from build123d import *

# Parameters (mm, degrees)
F0_R         = 12.7
F0_R_2       = 6.25
F1_DEPTH     = 4
F3_R         = 12.7
F4_DEPTH     = 3
F7_DEPTH     = 5.5
F10_DEPTH    = 3
F11_R        = 2.74999
F12_T1_DEPTH = 45.8363262896
F13_SIZE     = 2.54


# Not quite as in the source:
# - a fillet or chamfer that OpenCascade refuses, or shapes differently, is made with other operations: its cross-section is extruded or revolved along the edge and cut away or added
# - a fillet or chamfer is up to 0.001 mm smaller than in the source, because OpenCascade refuses the exact size


with BuildPart() as f1:
    # F0 (on Top) → F1 (new body)
    with BuildSketch(Plane.XY):
        Circle(F0_R)
        Circle(F0_R_2, mode=Mode.SUBTRACT)
    extrude(amount=F1_DEPTH)

    # F3 (on offset) → F4 (join)
    with BuildSketch(Plane.XY.offset(4)):
        Circle(F3_R)
    extrude(amount=F4_DEPTH)

    # F6 (on offset) → F7 (join)
    with BuildSketch(Plane.XY.offset(7)):
        with BuildLine():
            Line((3.67872e-05, 2.75), (12.3864002526, 2.75))
            ThreePointArc((12.3864002526, 2.75), (11.4283726358, 5.5236330803), (9.8540587351, 8))
            Line((9.8540587351, 8), (-9.8539683968, 8))
            ThreePointArc((-9.8539683968, 8), (-11.4266416959, 5.5228386705), (-12.3863266781, 2.75))
            Line((-12.3863266781, 2.75), (-4.0361126885, 2.75))
            Line((-4.0361126885, 2.75), (3.67872e-05, 2.75))
        make_face()
        with BuildLine():
            Line((12.3864002526, -2.75), (3.67872e-05, -2.75))
            Line((3.67872e-05, -2.75), (-4.0361126885, -2.75))
            Line((-4.0361126885, -2.75), (-12.3863266781, -2.75))
            ThreePointArc((-12.3863266781, -2.75), (-11.4266416959, -5.5228386705), (-9.8539683968, -8))
            Line((-9.8539683968, -8), (9.8540587351, -8))
            ThreePointArc((9.8540587351, -8), (11.4283726358, -5.5236330803), (12.3864002526, -2.75))
        make_face()
    extrude(amount=F7_DEPTH)

    # F9 (on offset) → F10 (join)
    with BuildSketch(Plane.XY.offset(12.5)):
        with BuildLine():
            Line((-9.8539683968, -8), (9.8540587351, -8))
            ThreePointArc((9.8540587351, -8), (12.7066576307, 0), (9.8540587351, 8))
            Line((9.8540587351, 8), (-9.8539683968, 8))
            ThreePointArc((-9.8539683968, 8), (-12.7123228833, 0), (-9.8539683968, -8))
        make_face()
    extrude(amount=F10_DEPTH)

    # F11 (radius 2.75 in the source; OpenCascade refuses exactly that, so slightly less here)
    f11_edges = [f1.edges().sort_by_distance(p)[0] for p in [
        (3.7e-05, -2.75, 7),
        (3.7e-05, -2.75, 12.5),
        (3.7e-05, 2.75, 12.5),
        (3.7e-05, 2.75, 7),
    ]]
    fillet(f11_edges, radius=F11_R)

    # F12: chamfer of 5.08 on 2 edges, made by hand

    # F12_s2 → F12_t1 (cut)
    with BuildSketch(Plane.YZ.offset(-22.9181179756)):
        Polygon((8, 10.42), (2.92, 15.5), (8, 15.5), align=None)
        Polygon((-8, 10.42), (-2.92, 15.5), (-8, 15.5), align=None)
    extrude(amount=F12_T1_DEPTH, mode=Mode.SUBTRACT)

    # F13
    f13_edges = [f1.edges().sort_by_distance(p)[0] for p in [
        (-0.002558, 2.92, 15.5),
        (-0.002558, -2.92, 15.5),
    ]]
    chamfer(f13_edges, length=F13_SIZE)


solid = f1.part
Verification items for the finished model (mm, model axes). A direction names the side the tool comes from. Coordinates: 2 decimals unless noted, no trailing zeros. Write each loop counter-clockwise with the first axis right and the second up, starting at its lowest first coordinate (ties: lowest second). Pieces come first, ordered by that corner, then holes. Notation, with made-up numbers: M 89,21 L 111,21 A4 ccw 111,25 Z; hole C 62,32 d3. An arc over 180 degrees is marked long. Use a Markdown table: item, result.
Q1. Thickness scan on line 1 (Y direction, x = 0, z = 0.85); line 2 (Z direction, x = -1, y = -2.5); line 3 (Y direction, x = -9.5, z = 11.5). Record the ranges inside material, lowest first.
Reply:
| item | result |
|---|---|
| line 1 | y = -12.7 to -6.25, 6.25 to 12.7 |
| line 2 | z = 4 to 8.6, 10.9 to 14.62 |
| line 3 | y = -6.92 to -2.12, 2.12 to 6.92 |
Q2. Set-up check for faces 1 (the face through (0, -8, 9)), 2 (the face through (0, 8, 9)), 3 (the face through (0.18, 1.92, 11.72)): record each of +Z, -Z, +X, -X, +Y, -Y from which the full face is reachable in a straight line by a thin tool's end or side.
Reply:
| item | result |
|---|---|
| face 1 | +Z, +X, -X, -Y |
| face 2 | +Z, +X, -X, +Y |
| face 3 | +X, -X |
Q3. Draft check along Z on faces 4 (the face through (-2.75, -12.4, 3.45)), 5 (the face through (-0.18, -1.92, 11.72)), 6 (the face through (-0.181, -2.518, 14.615)). Enter one of: +Z half, -Z half, draft (parallel to the pull), parting line (faces both ways), or undercut.
Reply:
| item | result |
|---|---|
| face 4 | draft |
| face 5 | undercut |
| face 6 | +Z half |
Q4. Sectioned sample at B-B, the plane z = 11. Record the boundary of the cut face in (x, y).
Reply:
| item | result |
|---|---|
| outline | M -12.45,-2.45 A12.65 ccw -10.3,-7.42 L 10.3,-7.42 A12.58 ccw 12.45,-2.45 Z; M -12.45,2.45 L 12.45,2.45 A12.58 ccw 10.3,7.42 L -10.3,7.42 A12.65 ccw Z |
Q5. Go/stop test with flat-tipped pins: P1, Ø12, axis at x = 3, y = 7, coming from the +Z side; P2, Ø2, axis at x = -1, y = -1.5, coming from the -Z side; P3, Ø10, axis at x = 9.5, y = -1, coming from the +Z side; P4, Ø2.5, axis at x = 2.5, z = 8.5, coming from the +Y side. Record where each tip stops, or that it passes through.
Reply:
| item | result |
|---|---|
| P1 | stops at z = 15.24 |
| P2 | stops at z = 4 |
| P3 | stops at z = 15.5 |
| P4 | stops at y = 8 |
Q6. Sectioned sample at D-D, the plane z = 8.5. Record the boundary of the cut face in (x, y), plus the area to 3 significant figures.
Reply:
| item | result |
|---|---|
| outline | M -12.45,-2.45 A12.65 ccw -9.85,-8 L 9.85,-8 A12.58 ccw 12.45,-2.45 Z; M -12.45,2.45 L 12.45,2.45 A12.58 ccw 9.85,8 L -9.85,8 A12.65 ccw Z |
| area | 254 mm² |
